For this review, take the finished solid that the model builds, in its own axes (mm). Give positions to 0.01 mm unless a question says otherwise; leave off trailing zeros. Order: outer loops, then holes, each group sorted by start corner. A loop starts at its lowest first (then second) coordinate and runs counter-clockwise, first axis right, second up. Notation, with made-up numbers: (56, -24.75) - (88, -24.75) arc R19 ccw to (88, 5.25) - close; hole circle Ø9 at (57, -17.75). An arc over 180 degrees is marked (long way). One line per item, written item: value.
```python
from build123d import *

# Parameters (mm, degrees)
SKETCH1_W           = 511.95
SKETCH1_H           = 300
SKETCH1_W_2         = 423.8
SKETCH1_H_2         = 161.9
BOSS_EXTRUDE1_DEPTH = 38.1
SHELL1_START        = -34.925
SHELL1_OUTLINE_W    = 430.15
SHELL1_OUTLINE_H    = 168.25
SHELL1_OUTLINE_W_2  = 518.3
SHELL1_OUTLINE_H_2  = 306.35
SHELL1_DEPTH        = 31.75


# Read off the part's stored shape, not the designer's step: Shell1
with BuildPart() as part:
    # Sketch1 → Boss-Extrude1 (new body)
    with BuildSketch(Plane.XY):
        Polygon((0, 0), (1850, 0), (1869.05, 0), (1869.05, 38.1), (1869.05, 238.1), (1369.05, 238.1), (1369.05, 38.1), (1069.1, 38.1), (1069.1, 338.1), (1069.1, 376.2), (0, 376.2), (0, 338.1), (80.95, 338.1), (80.95, 38.1), (0, 38.1), align=None)
        with Locations((775.025, 188.1)):
            Rectangle(SKETCH1_W, SKETCH1_H, mode=Mode.SUBTRACT)
        Polygon((451.617753988, 38.1), (119.05, 38.1), (119.05, 313.784791922), align=None, mode=Mode.SUBTRACT)
        Polygon((148.382246012, 338.1), (480.95, 338.1), (480.95, 62.415208078), align=None, mode=Mode.SUBTRACT)
        with Locations((1619.05, 119.05)):
            Rectangle(SKETCH1_W_2, SKETCH1_H_2, mode=Mode.SUBTRACT)
    extrude(amount=-BOSS_EXTRUDE1_DEPTH)

    # Shell1 outline → Shell1 (cut)
    with BuildSketch(Plane.XY.offset(SHELL1_START)):
        Polygon((84.125, 34.925), (3.175, 34.925), (3.175, 3.175), (1865.875, 3.175), (1865.875, 234.925), (1372.225, 234.925), (1372.225, 34.925), (1065.925, 34.925), (1065.925, 373.025), (3.175, 373.025), (3.175, 341.275), (84.125, 341.275), align=None)
        Polygon((460.42283517, 34.925), (115.875, 34.925), (115.875, 320.540779362), align=None, mode=Mode.SUBTRACT)
        with Locations((1619.05, 119.05)):
            Rectangle(SHELL1_OUTLINE_W, SHELL1_OUTLINE_H, mode=Mode.SUBTRACT)
        Polygon((139.57716483, 341.275), (484.125, 341.275), (484.125, 55.659220638), align=None, mode=Mode.SUBTRACT)
        with Locations((775.025, 188.1)):
            Rectangle(SHELL1_OUTLINE_W_2, SHELL1_OUTLINE_H_2, mode=Mode.SUBTRACT)
    extrude(amount=SHELL1_DEPTH, mode=Mode.SUBTRACT)


solid = part.part
```
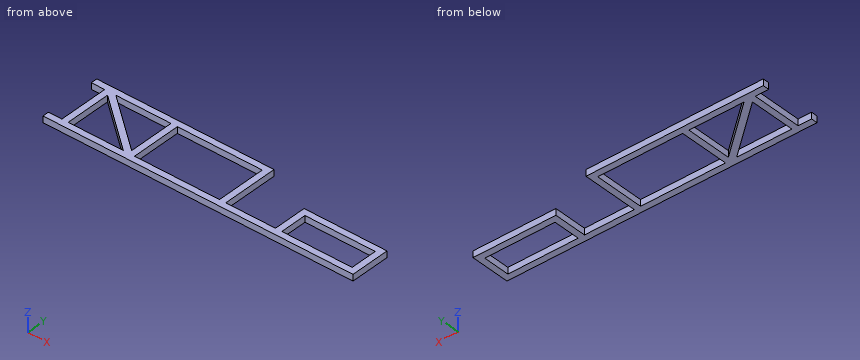
(1) Wall thickness on line 1 (Y direction, x = 1787, z = -10.5) (3 decimals); line 2 (Y direction, x = 959.5, z = -33.5) (3 decimals); line 3 (Y direction, x = 1277.5, z = -26.5) (3 decimals): over which ranges is each line inside the solid? List them lowest first. Write a range as from..to.
Answers below:
line 1: y = 0..3.175, 34.925..38.1, 200..203.175, 234.925..238.1
line 2: y = 0..3.175, 34.925..38.1, 338.1..341.275, 373.025..376.2
line 3: y = 0..3.175, 34.925..38.1
(2) Take a section at C-C (z = -13.5). Give the number of separate pieces and of enclosed holes in the cut face, then the cut area to 3 significant figures.
Answers below:
separate pieces: 5
enclosed holes: 5
area: 31,700 mm^2
(3) Take a section at A-A (x = 287.5). Write out the cut boundary in (y, z) (3 decimals), then the cut area to 3 significant figures.
Answers below:
outline: (0, -38.1) - (38.1, -38.1) - (38.1, 0) - (0, 0) - close; (174.147, -38.1) - (222.777, -38.1) - (222.777, 0) - (174.147, 0) - close; (338.1, -38.1) - (376.2, -38.1) - (376.2, 0) - (338.1, 0) - close; hole (3.175, -34.925) - (34.925, -34.925) - (34.925, -3.175) - (3.175, -3.175) - close; hole (178.271, -34.925) - (218.653, -34.925) - (218.653, -3.175) - (178.271, -3.175) - close; hole (341.275, -34.925) - (373.025, -34.925) - (373.025, -3.175) - (341.275, -3.175) - close
area: 1,460 mm^2
(4) For P1, Ø5, axis at y = 118.5, z = -5.5, coming from the -X side, flat-tipped, find the tip position at first contact; note if it passes through.
Answers below:
P1: stops at x = 80.95
(5) Take a section at B-B (x = 1643.5). Write out the cut boundary in (y, z) (3 decimals).
Answers below:
outline: (0, -38.1) - (38.1, -38.1) - (38.1, 0) - (0, 0) - close; (200, -38.1) - (238.1, -38.1) - (238.1, 0) - (200, 0) - close; hole (3.175, -34.925) - (34.925, -34.925) - (34.925, -3.175) - (3.175, -3.175) - close; hole (203.175, -34.925) - (234.925, -34.925) - (234.925, -3.175) - (203.175, -3.175) - close
